Build history of the part. All positions in model axes, mm. A direction names the side the tool comes from. Round coordinates to 2 decimals unless told otherwise and drop trailing zeros. Loops run counter-clockwise (first coordinate to the right, second up) from the corner with the lowest first, then second, coordinate; pieces in that order, holes last. Notation, with made-up numbers: (-10, 5) - (37, 5) arc R18 ccw to (37, 33) - close; hole circle Ø10 at (-3, 39). An arc over 180 degrees is marked (long way). Use a Markdown table: item, result.
from build123d import *

# Parameters (mm, degrees)
F1_DEPTH = 20
F2_R     = 3
F3_R     = 2
F4_R     = 5
F6_D     = 2.8
F6_DEPTH = 10
F6_TIP   = 0.8412048666
F7_R     = 2


with BuildPart() as f1:
    # F0 (on Right) → F1 (new body)
    with BuildSketch(Plane.YZ):
        Polygon((11.7727210118, 5), (11.7727210118, 0), (21.7727210118, 0), (21.7727210118, 20), (-52.7272789882, 20), (-52.7272789882, -34.9435843527), (-41.7272789882, -35), (-41.7272789882, 15), (16.7727210118, 15), (16.7727210118, 5), align=None)
    extrude(amount=F1_DEPTH)

    # F2
    f2_edges = [f1.edges().sort_by_distance(p)[0] for p in [
        (10, 21.772721, 20),
        (10, 21.772721, 0),
    ]]
    fillet(f2_edges, radius=F2_R)

    # F3
    f3_edges = [f1.edges().sort_by_distance(p)[0] for p in [
        (10, -41.727279, 15),
        (10, 16.772721, 15),
    ]]
    fillet(f3_edges, radius=F3_R)

    # F4
    f4_edges = [f1.edges().sort_by_distance(p)[0] for p in [
        (10, -52.727279, -34.943584),
        (10, -52.727279, 20),
    ]]
    fillet(f4_edges, radius=F4_R)

    # F6
    with Locations(Plane(origin=(0, -41.7272789882, 0), x_dir=(-1, 0, 0), z_dir=(0, 1, 0))):
        with Locations((-10, -28), (-10, -10)):
            Hole(F6_D / 2, depth=F6_DEPTH)
            with Locations((0, 0, -(F6_DEPTH + F6_TIP / 2))):  # 118° drill point
                Cone(0, F6_D / 2, F6_TIP, mode=Mode.SUBTRACT)

    # F7
    f7_edges = [f1.edges().sort_by_distance(p)[0] for p in [
        (0, -52.727279, -7.484581),
        (20, -14.477279, 20),
    ]]
    fillet(f7_edges, radius=F7_R)


solid = f1.part
Q1. Drop flat-ended pins along their axis: pin 1 (4 mm diameter, centred on x = 13.5, y = 8, fed in from -Z); pin 2 (2 mm diameter, centred on x = 7.5, y = 16.5, fed in from -Z); pin 3 (4 mm diameter, centred on x = 17.5, z = -14.5, fed in from +Y). Give the stop position or say it passes through.
Results found:
| item | result |
|---|---|
| pin 1 | stops at z = 15 |
| pin 2 | stops at z = 0 |
| pin 3 | stops at y = -41.73 |
Q2. Probe line 1 (Z direction, x = 10, y = -44); line 2 (Y direction, x = 9.25, z = 11); line 3 (Z direction, x = 1.75, y = 15). List the from-to ranges inside material, lowest first.
Results found:
| item | result |
|---|---|
| line 1 | z = -34.99 to -29.4, -26.6 to -11.4, -8.6 to 20 |
| line 2 | y = -52.73 to -41.73, 16.77 to 21.77 |
| line 3 | z = 0.02 to 5, 14.99 to 19.98 |
Q3. Pull direction Z, two halves, no side cores. Call faces 4 (the face through (10, 16.773, 9)), 5 (the face through (20, -42, -2)), 6 (the face through (19.4, -14.94, 19.43)), 7 (the face through (10.14, -41.126, 14.43)): pulls with the +Z half, pulls with the -Z half, needs draft (parallel to the pull), parting line crosses it, or undercut.
Results found:
| item | result |
|---|---|
| face 4 | undercut |
| face 5 | needs draft |
| face 6 | pulls with the +Z half |
| face 7 | pulls with the -Z half |
Q4. Cut at A-A, the plane z = 11. List the corners of the cut face in (x, y), plus the area to 3 significant figures.
Results found:
| item | result |
|---|---|
| outline | (0, -50.73) arc R2 ccw to (2, -52.73) - (18, -52.73) arc R2 ccw to (20, -50.73) - (20, -41.73) - (0, -41.73) - close; (0, 16.77) - (20, 16.77) - (20, 19.77) arc R2 ccw to (18, 21.77) - (2, 21.77) arc R2 ccw to (0, 19.77) - close |
| area | 317 mm2 |
Q5. Cut at B-B, the plane x = 16.75. List the corners of the cut face in (y, z), plus the area to 3 significant figures.
Results found:
| item | result |
|---|---|
| outline | (-52.73, -29.97) arc R5 ccw to (-47.75, -34.97) - (-41.73, -35) - (-41.73, 13) arc R2 cw to (-39.73, 15) - (14.77, 15) arc R2 cw to (16.77, 13) - (16.77, 5) - (11.77, 5) - (11.77, 0) - (18.77, 0) arc R3 ccw to (21.77, 3) - (21.77, 17) arc R3 ccw to (18.77, 20) - (-47.73, 20) arc R5 ccw to (-52.73, 15) - close |
| area | 1,010 mm2 |
Q6. Cut at D-D, the plane y = -36. List the corners of the cut face in (x, z), plus the area to 3 significant figures.
Results found:
| item | result |
|---|---|
| outline | (0, 15) - (20, 15) - (20, 18) arc R2 ccw to (18, 20) - (2, 20) arc R2 ccw to (0, 18) - close |
| area | 98.3 mm2 |
Q7. Cut at C-C, the plane z = -1.5. List the corners of the cut face in (x, y).
Results found:
| item | result |
|---|---|
| outline | (0, -50.73) arc R2 ccw to (2, -52.73) - (18, -52.73) arc R2 ccw to (20, -50.73) - (20, -41.73) - (0, -41.73) - close |
Q8. Which spindle directions (+Z, -Z, +X, -X, +Y, -Y) get a long thin tool onto all of the face, cutting with end or side? Do faces 1 (the face through (10, 11.773, 3)), 2 (the face through (10.112, 20.917, 19.098)), 3 (the face through (8.6, -46.8, -27.94)). Say none if no direction does.
Results found:
| item | result |
|---|---|
| face 1 | -Z, +X, -X |
| face 2 | +Z, +X, -X, +Y |
| face 3 | +Y |
